from build123d import *

# Parameters (mm, degrees)
BOSS_EXTRU_1_DEPTH      = 8
ENL_V_MAT_EXTRU_1_REACH = 45.749
ESQUISSE2_R             = 1
D_GAGEMENT_M21_D        = 2.4
D_GAGEMENT_M21_DEPTH    = 11
D_GAGEMENT_M21_TIP      = 0.721032743
CONG_1_R                = 2
ESQUISSE5_R             = 7.5
BOSS_EXTRU_2_DEPTH      = 10
ESQUISSE6_R             = 1
ENL_V_MAT_EXTRU_2_DEPTH = 6
ESQUISSE8_R             = 3.5
ENL_V_MAT_EXTRU_3_DEPTH = 18


with BuildPart() as part:
    # Esquisse1 → Boss.-Extru.1 (new body)
    with BuildSketch(Plane.XY):
        with BuildLine():
            Line((21, -6.417424305), (27, -6.417424305))
            Line((27, -6.417424305), (27, -25))
            Line((27, -25), (35, -25))
            Line((35, -25), (35, -28.4))
            Line((35, -28.4), (26, -28.4))
            Line((26, -28.4), (26, -32.6))
            Line((26, -32.6), (35, -32.6))
            Line((35, -32.6), (35, -36))
            Line((35, -36), (21, -36))
            Line((21, -36), (21, -15.582575695))
            ThreePointArc((21, -15.582575695), (0, -11), (21, -6.417424305))
        make_face()
    extrude(amount=BOSS_EXTRU_1_DEPTH)

    # Enlèv. mat.-Extru.1: up to this face of the body (flat: up to its plane)
    enl_v_mat_extru_1_end = Plane(part.part.faces().sort_by_distance((28, -36, 4))[0])
    # Esquisse2 → Enlèv. mat.-Extru.1 (cut, up to the picked face)
    with BuildSketch(Plane(origin=(0, -25, 0), x_dir=(1, 0, 0), z_dir=(0, 1, 0)), mode=Mode.PRIVATE) as enl_v_mat_extru_1_sk1:
        with Locations(Location((30, -4, 0), (0, 0, 270))):
            Circle(ESQUISSE2_R)
    enl_v_mat_extru_1_tool1 = split(extrude(enl_v_mat_extru_1_sk1.sketch, amount=-ENL_V_MAT_EXTRU_1_REACH, mode=Mode.PRIVATE), bisect_by=enl_v_mat_extru_1_end, keep=Keep.BOTH, mode=Mode.PRIVATE)
    add(enl_v_mat_extru_1_tool1.solids().sort_by(Axis((30, -25, 4), (0, -1, 0)))[0], mode=Mode.SUBTRACT)

    # Dégagement M21
    with Locations(Plane(origin=(0, -25, 0), x_dir=(1, 0, 0), z_dir=(0, 1, 0))):
        with Locations((30, -4)):
            Hole(D_GAGEMENT_M21_D / 2, depth=D_GAGEMENT_M21_DEPTH)
            with Locations((0, 0, -(D_GAGEMENT_M21_DEPTH + D_GAGEMENT_M21_TIP / 2))):  # 118° drill point
                Cone(0, D_GAGEMENT_M21_D / 2, D_GAGEMENT_M21_TIP, mode=Mode.SUBTRACT)

    # Congé1
    cong_1_edges = [part.edges().sort_by_distance(p)[0] for p in [
        (21, -36, 4),
        (21, -6.417424305, 4),
        (27, -6.417424305, 4),
    ]]
    fillet(cong_1_edges, radius=CONG_1_R)

    # Esquisse5 → Boss.-Extru.2 (add)
    with BuildSketch(Plane.XY.offset(8)):
        with Locations((11, -11)):
            Circle(ESQUISSE5_R)
    extrude(amount=BOSS_EXTRU_2_DEPTH)

    # Esquisse6 → Enlèv. mat.-Extru.2 (cut)
    with BuildSketch(Plane(origin=(0, 0, 0), x_dir=(-1, 0, 0), z_dir=(0, 0, -1))):
        with Locations((-11, -3.5)):
            Circle(ESQUISSE6_R)
        with Locations((-11, -18.5)):
            Circle(ESQUISSE6_R)
    extrude(amount=-ENL_V_MAT_EXTRU_2_DEPTH, mode=Mode.SUBTRACT)

    # Esquisse8 → Enlèv. mat.-Extru.3 (cut)
    with BuildSketch(Plane(origin=(0, 0, 0), x_dir=(-1, 0, 0), z_dir=(0, 0, -1))):
        with Locations((-11, -11)):
            Circle(ESQUISSE8_R)
    extrude(amount=-ENL_V_MAT_EXTRU_3_DEPTH, mode=Mode.SUBTRACT)


solid = part.part
Can you work these out from the model? Positions are in its coordinate system, mm. A direction names the side the tool comes from. Give positions to 0.01 mm unless a question says otherwise; leave off trailing zeros. Write each loop counter-clockwise with the first axis right and the second up, starting at its lowest first coordinate (ties: lowest second). Pieces come first, ordered by that corner, then holes. Notation, with made-up numbers: (41.5, 25.25) -> (91.5, 25.25) arc R26 ccw to (91.5, 40.25) -> close; hole circle Ø7 at (-26.5, 9.25). An arc over 180 degrees is marked (long way). Answer as a JSON object with one key per item and string values. Group by question number.
Item 1: Please list where these lines run through material, in increasing order: line 1 (Y direction, x = 11, z = 4.75); line 2 (X direction, y = -33.55, z = 4); line 3 (Z direction, x = 30, y = -35). Write a range as [from, to].
Item 2: I'm going to push flat-ended pins straight in: P1, Ø11, axis at x = 11, y = -11, coming from the +Z side; P2, Ø1, axis at x = 21.5, z = 2, coming from the +Y side; P3, Ø0.6, axis at x = 11, y = -18.5, coming from the -Z side; P4, Ø8, axis at x = 16, z = 11, coming from the +Y side. Where does each tip first touch, or does it pass through?
Item 3: We'd pull the mould along Y, two halves only. Please class faces 5 (the face through (11.8, -4.1, 3)), 6 (the face through (35, -27, 4)), 7 (the face through (11, -3, 6)), 8 (the face through (26.4, -6.99, 4.06)): +Y half, -Y half, draft (parallel to the pull), parting line (faces both ways), or undercut.
Item 4: Suppose I cut it at A-A (x = 30). Please give me the cut outline in (y, z), plus the area to 3 significant figures.
Item 5: Suppose I cut it at D-D (y = -11). Please give me the cut outline in (x, z), plus the area to 3 significant figures.
Item 6: Suppose I cut it at C-C (x = 11). Please give me the cut outline in (y, z).
Item 7: For faces 1 (the face through (11, -18, 6)), 2 (the face through (24, -6.417, 4)), 3 (the face through (32, -28.4, 4)), 4 (the face through (9.37, -18.32, 12.93)), which set-ups out of +Z, -Z, +X, -X, +Y, -Y let a thin tool reach every point of the face, with its end or its side?
Item 8: Suppose I cut it at B-B (z = 4). Please give me the cut outline in (x, y).
Findings:
{
 "1": {"line 1": "y = [-22, -19.5], [-17.5, -14.5], [-7.5, -4.5], [-2.5, 0]", "line 2": "x = [21, 28.8], [31.2, 35]", "line 3": "z = [0, 2.8], [5.2, 8]"},
 "2": {"P1": "stops at z = 18", "P2": "stops at y = -6.01", "P3": "stops at z = 6", "P4": "stops at y = -0.25"},
 "3": {"face 5": "undercut", "face 6": "draft", "face 7": "undercut", "face 8": "+Y half"},
 "4": {"outline": "(-36, 0) -> (-32.6, 0) -> (-32.6, 2.8) -> (-36, 2.8) -> close; (-36, 5.2) -> (-32.6, 5.2) -> (-32.6, 8) -> (-36, 8) -> close; (-28.4, 0) -> (-25, 0) -> (-25, 2.8) -> (-28.4, 2.8) -> close; (-28.4, 5.2) -> (-25, 5.2) -> (-25, 8) -> (-28.4, 8) -> close", "area": "38.1 mm²"},
 "5": {"outline": "(0, 0) -> (7.5, 0) -> (7.5, 18) -> (3.5, 18) -> (3.5, 8) -> (0, 8) -> close; (14.5, 0) -> (27, 0) -> (27, 8) -> (18.5, 8) -> (18.5, 18) -> (14.5, 18) -> close", "area": "240 mm²"},
 "6": {"outline": "(-22, 0) -> (-19.5, 0) -> (-19.5, 6) -> (-17.5, 6) -> (-17.5, 0) -> (-14.5, 0) -> (-14.5, 18) -> (-18.5, 18) -> (-18.5, 8) -> (-22, 8) -> close; (-7.5, 0) -> (-4.5, 0) -> (-4.5, 6) -> (-2.5, 6) -> (-2.5, 0) -> (0, 0) -> (0, 8) -> (-3.5, 8) -> (-3.5, 18) -> (-7.5, 18) -> close"},
 "7": {"face 1": "-Z", "face 2": "+Z, -Z, +X, +Y", "face 3": "+Z, -Z, +X", "face 4": "+Z"},
 "8": {"outline": "(20.49, -5.43) arc R11 ccw (long way) to (21, -15.58) -> (21, -34) arc R2 ccw to (23, -36) -> (28.8, -36) -> (28.8, -32.6) -> (26, -32.6) -> (26, -28.4) -> (28.8, -28.4) -> (28.8, -25) -> (27, -25) -> (27, -8.42) arc R2 ccw to (25, -6.42) -> (22.21, -6.42) arc R2 cw to start; (31.2, -36) -> (35, -36) -> (35, -32.6) -> (31.2, -32.6) -> close; (31.2, -28.4) -> (35, -28.4) -> (35, -25) -> (31.2, -25) -> close; hole circle Ø7 at (11, -11); hole circle Ø2 at (11, -18.5); hole circle Ø2 at (11, -3.5)"}
}
